Autodesk Inventor part; units mm, degrees
ref_plane "YZ Plane" through (0, 0, 0) normal (1, 0, 0) x (0, 1, 0)
ref_plane "XZ Plane" through (0, 0, 0) normal (0, 1, 0) x (-1, 0, 0)
ref_plane "XY Plane" through (0, 0, 0) normal (0, 0, 1) x (1, 0, 0)
sketch "Sketch1" plane through (0, 0, 0) normal (0, 1, 0) x (-1, 0, 0)
  line L0 (0, 0) -> (25.4, 0)
  line L1 (25.4, 0) -> (25.4, -50.8)
  line L2 (25.4, -50.8) -> (0, -50.8)
  line L3 (0, -50.8) -> (0, 0)
  line L4 (3.175, -3.175) -> (22.225, -3.175)
  line L5 (22.225, -3.175) -> (22.225, -47.625)
  line L6 (22.225, -47.625) -> (3.175, -47.625)
  line L7 (3.175, -47.625) -> (3.175, -3.175)
  dimension "d0" = 25.4
  dimension "d1" = 50.8
  dimension "d2" = 3.175
extrude "Extrusion1" add sketch "Sketch1" along normal blind 711.2
sketch "Sketch2" plane through (-25.4, 0, -50.8) normal (-1, 0, 0) x (0, 0, 1)
  circle A0 centre (28.575, 355.6) radius 4.7625
  line L0 (0, 711.2) -> (50.8, 711.2)
  line L1 (0, 0) -> (0, 711.2)
  circle A1 centre (12.7, 622.3) radius 4.7625
  line L2 (50.8, 0) -> (50.8, 711.2)
  circle A2 centre (12.7, 88.9) radius 4.7625
  line L3 (0, 88.9) -> (50.8, 88.9) construction
  line L4 (50.8, 0) -> (50.8, 711.2)
  line L5 (0, 622.3) -> (50.8, 622.3) construction
  circle A3 centre (25.4, 177.8) radius 3.3734
  line L6 (50.8, 0) -> (0, 0)
  circle A4 centre (25.4, 241.3) radius 3.3734
  circle A5 centre (25.4, 533.4) radius 3.3734
  circle A6 centre (25.4, 469.9) radius 3.3734
  circle A7 centre (12.7, 254) radius 3.3734
  circle A8 centre (38.1, 279.4) radius 3.3734
  dimension "d6" = 355.6
  dimension "d7" = 28.575
  dimension "d10" = 9.525
  dimension "d11" = 38.1
  dimension "d14" = 38.1
  dimension "d16" = 266.7
  dimension "d17" = 266.7
  dimension "d18" = 6.7469
  dimension "d19" = 25.4
  dimension "d20" = 177.8
  dimension "d22" = 241.3
  dimension "d23" = 25.4
  dimension "d25" = 25.4
  dimension "d26" = 177.8
  dimension "d28" = 25.4
  dimension "d29" = 241.3
  dimension "d30" = 6.7469
  dimension "d31" = 6.7469
  dimension "d32" = 12.7
  dimension "d33" = 12.7
  dimension "d34" = 25.4
  dimension "d35" = 38.1
  dimension "d38" = 63.5
extrude "Extrusion2" cut sketch "Sketch2" against normal blind 25.4 contours A0 | A1 | A2 | A3 | A4 | A5 | A6
extrude "Extrusion3" cut sketch "Sketch2" against normal blind 25.4 contours A7 | A8
properties part number "1x2x28" material "Aluminum 6061"
Geometry: final body of the model. Coordinates: model frame, mm. A direction names the side the tool comes from. Give positions to 0.01 mm unless a question says otherwise; leave off trailing zeros. Write each loop counter-clockwise with the first axis right and the second up, starting at its lowest first coordinate (ties: lowest second). Pieces come first, ordered by that corner, then holes. Notation, with made-up numbers: (-36, 81.25) - (-32, 81.25) arc R18 ccw to (-32, 109.25) - close; hole circle Ø2 at (79.5, 55.5). An arc over 180 degrees is marked (long way). Return JSON: item names as keys, results as strings. Group by question number.
1) Section B-B on y = 596. Return the cut outline in (x, z) (3 decimals), plus the area to 3 significant figures.
2) Section A-A on x = -7.5. Return the cut outline in (y, z) (3 decimals).
3) Mould query, pull axis X, two halves, no side actions, for faces 1 (the flat face through (-22.225, 351, -25)), 2 (the flat face through (-3.175, 351, -26)), 3 (the flat face through (-2, 0, -27)), 4 (the flat face through (0, 351, -26)). Classes: released by +X, released by -X, zero draft, split by the parting line, or undercut.
4) Set-up query: faces 5 (the flat face through (-2, 711.2, -27)), 6 (the flat face through (-13, 351, -47.625)). Return all of +Z, -Z, +X, -X, +Y, -Y with unobstructed straight access to the full face (end or side cutting, diameter ignored); none if empty.
5) Line query: line 1 (Y direction, x = -23.5, z = -38.1); line 2 (Z direction, x = -15.5, y = 190) (3 decimals); line 3 (Y direction, x = -0.9, z = -25.4). Output: solid intervals per line, ascending.
6) First-contact query: P1, Ø12, axis at y = 207.5, z = -18.5, coming from the +X side. Flat tip, straight axial feed; report the tip coordinate or a pass-through.
Filled in:
{
 "1": {"outline": "(-25.4, -50.8) - (0, -50.8) - (0, 0) - (-25.4, 0) - close; hole (-22.225, -47.625) - (-3.175, -47.625) - (-3.175, -3.175) - (-22.225, -3.175) - close", "area": "444 mm^2"},
 "2": {"outline": "(0, -50.8) - (711.2, -50.8) - (711.2, -47.625) - (0, -47.625) - close; (0, -3.175) - (711.2, -3.175) - (711.2, 0) - (0, 0) - close"},
 "3": {"face 1": "undercut", "face 2": "undercut", "face 3": "zero draft", "face 4": "released by +X"},
 "4": {"face 5": "+Z, -Z, +X, -X, +Y", "face 6": "+Y, -Y"},
 "5": {"line 1": "y = 0 to 84.14, 93.66 to 250.63, 257.37 to 617.54, 627.06 to 711.2", "line 2": "z = -50.8 to -47.625, -3.175 to 0", "line 3": "y = 0 to 174.43, 181.17 to 237.93, 244.67 to 352.05, 359.15 to 466.53, 473.27 to 530.03, 536.77 to 711.2"},
 "6": {"P1": "stops at x = 0"}
}
